Can you work these out from the model? Positions are in its coordinate system, mm. A direction names the side the tool comes from. Give positions to 0.01 mm unless a question says otherwise; leave off trailing zeros.
Autodesk Inventor part; units mm, degrees
ref_plane "YZ Plane" through (0, 0, 0) normal (1, 0, 0) x (0, 1, 0)
ref_plane "XZ Plane" through (0, 0, 0) normal (0, 1, 0) x (-1, 0, 0)
ref_plane "XY Plane" through (0, 0, 0) normal (0, 0, 1) x (1, 0, 0)
sketch "Szkic1" plane through (0, 0, 0) normal (0, 0, 1) x (1, 0, 0)
  circle A0 centre (0, 0) radius 4
  circle A1 centre (0, 0) radius 12.5 construction
  line L0 (0, 0) -> (-34.641, 20) construction
  line L1 (-44.641, 20) -> (-84.641, 20) construction
  line L2 (-34.641, 20) -> (-34.641, 30) construction
  line L3 (-34.641, 30) -> (5.2954, 11.3229)
  line L4 (-34.641, 20) -> (-34.641, 12) construction
  line L5 (-34.641, 12) -> (-7.8737, -9.7085)
  line L6 (-84.641, 20) -> (-84.641, 30)
  line L7 (-84.641, 30) -> (-34.641, 30)
  line L8 (-34.641, 12) -> (-39.641, 12)
  line L9 (-39.641, 12) -> (-39.641, 15) construction
  line L10 (-39.641, 20) -> (-34.641, 30) construction
  line L11 (-42.641, 20) -> (-37.641, 30) construction
  arc A2 (-1.3611, 14.436) -> (-13.5811, -5.0798) centre (0, 0) ccw
  line L12 (-104.0692, 0) -> (31.9282, 0) construction
  line L13 (-20.4848, 0.5192) -> (-10.0924, 18.5194) construction
  line L14 (-39.641, 12) -> (-44.641, 12)
  line L15 (-44.641, 12) -> (-44.641, 15)
  line L16 (-44.641, 15) -> (-39.641, 15) construction
  arc A3 (-39.641, 15) -> (-44.641, 20) centre (-44.641, 15) ccw
  arc A4 (-39.641, 15) -> (-36.641, 12) centre (-36.641, 15) ccw
  circle A5 centre (-76.641, 25) radius 0.75
  circle A6 centre (-69.641, 25) radius 0.75
  line L17 (-76.641, 25) -> (-69.641, 25) construction
  circle A7 centre (-59.641, 25) radius 0.75
  circle A8 centre (-49.641, 25) radius 0.75
  line L18 (-44.641, 20) -> (-44.641, 30)
  line L19 (-44.641, 15) -> (-44.641, 20)
  circle A9 centre (-16.4545, 9.5) radius 0.8
  circle A10 centre (-22.5167, 13) radius 0.8
  circle A11 centre (-34.641, 20) radius 0.8
  dimension "d0" = 25
  dimension "d1" = 29
  dimension "d2" = 8
  dimension "d4" = 40
  dimension "d5" = 30
  dimension "d6" = 50
  dimension "d7" = 10
  dimension "d8" = 5
  dimension "d9" = 3
  dimension "d10" = 8
  dimension "d11" = 22
  dimension "d16" = 5
  dimension "d17" = 3
  dimension "d20" = 5
  dimension "d21" = 3
  dimension "d23" = 1.5
  dimension "d24" = 1.5
  dimension "d25" = 8
  dimension "d26" = 5
  dimension "d27" = 15
  dimension "d31" = 10
  dimension "d43" = 1.6
  dimension "d45" = 19
  dimension "d46" = 7
extrude "Wyciągnięcie proste3" add sketch "Szkic1" along normal blind 6 contours L3 A2 L5 L8 A4 A3 L18 L7 | A3 A4 L8 L14 L15 L19
fillet "Zaokrąglenie4" radius 5 1 edges at (-34.641, 30, 3)
fillet "Zaokrąglenie6" radius 3 2 edges at (-44.641, 12, 3) (-34.641, 12, 3)
fillet "Zaokrąglenie8" radius 3 9 edges at (-34.6675, 29.8809, 6) (-40.1967, 30, 6) (-44.641, 30, 3) (-17.4977, 21.9826, 6) (-43.7623, 12.8787, 6) (-38.6728, 12, 6) (-34.7022, 11.8276, 6) (-23.698, 3.1251, 6) (-44.641, 22.5, 6)
properties part number "palec2" material "PLA"
1) If we mould it in two halves opening along Y, with no side actions, what happens to faces 4 (the face through (-12.387, 7.537, 2.958)), 5 (the face through (-44.641, 21, 1)), 6 (the face through (-23.84, 3.24, 1.48))? For each: +Y half, -Y half, draft (parallel to the pull), parting line (faces both ways), or undercut.
Values follow:
face 4: undercut
face 5: draft
face 6: -Y half
2) For pin 1 Ø1.5 at (x, y) = (-13, 18) entering from -Z; pin 2 Ø1.5 at (x, z) = (-38.5, 2) entering from -Y; pin 3 Ø2 at (x, z) = (-17, 2.5) entering from +Y; pin 4 Ø1.5 at (y, z) = (15.5, 2) entering from +X, each with a flat end and sliding along its axis, tell me the tip position at first contact or that it passes through.
Values follow:
pin 1: stops at z = 0
pin 2: stops at y = 12
pin 3: stops at y = 22.22
pin 4: stops at x = -2.03
3) For faces 1 (the face through (-38.63, 12.9, 5.14)), 2 (the face through (-39, 12, 1)), 3 (the face through (-17.044, 8.959, 2.958)), which set-ups out of +Z, -Z, +X, -X, +Y, -Y let a thin tool reach every point of the face, with its end or its side?
Values follow:
face 1: +Z, -X, -Y
face 2: +Z, -Z, -X, -Y
face 3: +Z, -Z
4) Please list where these lines run through material, in increasing order: L1, parallel to Y at x = -36, z = 2.25; L2, parallel to X at y = 19.5, z = 2.25; L3, parallel to Y at x = -6, z = 1.75.
Values follow:
L1: y = 12 to 30
L2: x = -44.64 to -35.27, -34.02 to -12.19
L3: y = 13.2 to 16.61
5) Suppose I cut it at A-A on z = 5. State how many separate pieces and enclosed holes the cut face has, plus the area to 3 significant figures.
Values follow:
separate pieces: 1
enclosed holes: 3
area: 614 mm2
